Source: CAD feature listing. Evaluate the final solid. Frame: model axes, mm. A direction names the side the tool comes from. Give positions to 0.01 mm unless a question says otherwise; leave off trailing zeros. Loops run counter-clockwise (first coordinate to the right, second up) from the corner with the lowest first, then second, coordinate; pieces in that order, holes last.
```python
from build123d import *

# Parameters (mm, degrees)
F1_DEPTH = 6.35


with BuildPart() as f1:
    # F0 (on Top) → F1 (new body, symmetric)
    with BuildSketch(Plane.XY):
        Polygon((-44.789236, 14.552905), (-40.419224, 17.727905), (-54.301441, 17.727905), (-43.082257, 9.299362), align=None)
        Polygon((-27.68127, -38.1), (-18.27958, -5.362784), (-44.789236, 14.552905), (-43.082257, 9.299362), (-21.934765, -6.587938), (-29.434755, -32.703328), align=None)
        Polygon((-12.292903, 14.552905), (0, 47.09419), (-4.677891, 43.695503), (-14.487496, 17.727905), (-40.419224, 17.727905), (-44.789236, 14.552905), align=None)
        Polygon((-4.677891, 43.695503), (0, 47.09419), (4.677891, 43.695503), (0, 56.078631), align=None)
        Polygon((4.677891, 43.695503), (0, 47.09419), (12.292903, 14.552905), (44.789236, 14.552905), (40.419224, 17.727905), (14.487496, 17.727905), align=None)
        Polygon((54.560881, 17.727905), (40.419224, 17.727905), (44.789236, 14.552905), (43.12004, 9.415647), align=None)
        Polygon((43.12004, 9.415647), (44.789236, 14.552905), (18.49915, -4.547961), (27.68127, -38.1), (29.468066, -32.600809), (22.140832, -5.82664), align=None)
        Polygon((29.468066, -32.600809), (27.68127, -38.1), (22.080786, -38.1), (33.036342, -45.639515), align=None)
        Polygon((27.68127, -38.1), (0, -19.05), (-27.68127, -38.1), (-22.080786, -38.1), (0, -22.904203), (22.080786, -38.1), align=None)
        Polygon((-22.080786, -38.1), (-27.68127, -38.1), (-29.434755, -32.703328), (-33.177816, -45.736876), align=None)
    extrude(amount=F1_DEPTH, both=True)


solid = f1.part
```
(1) Section D-D, the plane x = -24. Return the cut outline in (y, z), then the cut area to 3 significant figures.
A:
outline: (-39.42, -6.35) - (-35.57, -6.35) - (-35.57, 6.35) - (-39.42, 6.35) - close; (-25.28, -6.35) - (-13.78, -6.35) - (-13.78, 6.35) - (-25.28, 6.35) - close; (-5.04, -6.35) - (-1.07, -6.35) - (-1.07, 6.35) - (-5.04, 6.35) - close; (14.55, -6.35) - (17.73, -6.35) - (17.73, 6.35) - (14.55, 6.35) - close
area: 286 mm2
(2) First-contact query: pin 1 (1 mm diameter, centred on y = 22, z = -3.5, fed in from -X); pin 2 (2 mm diameter, centred on x = 42.5, z = -0.5, fed in from +Y). Flat tips, straight axial feed; report the tip coordinate or a pass-through.
A:
pin 1: stops at x = -13.06
pin 2: stops at y = 17.73
(3) Mould query, pull axis Y, two halves, no side actions, for faces 1 (the flat face through (12, 17, -6.35)), 2 (the flat face through (-31.349, 4.456, 0.089)), 3 (the flat face through (35, 17.728, 0)). Classes: pulls with the +Y half, pulls with the -Y half, needs draft (parallel to the pull), parting line crosses it, or undercut.
A:
face 1: needs draft
face 2: undercut
face 3: pulls with the +Y half
(4) Section C-C, the plane y = 6. Return the cut outline in (x, z).
A:
outline: (-38.69, -6.35) - (-33.4, -6.35) - (-33.4, 6.35) - (-38.69, 6.35) - close; (33.02, -6.35) - (38.42, -6.35) - (38.42, 6.35) - (33.02, 6.35) - close
(5) Section A-A, the plane z = -4. Return the cut outline in (x, y).
A:
outline: (-54.3, 17.73) - (-21.93, -6.59) - (-33.18, -45.74) - (0, -22.9) - (33.04, -45.64) - (22.14, -5.83) - (54.56, 17.73) - (14.49, 17.73) - (0, 56.08) - (-14.49, 17.73) - close; hole (-44.79, 14.55) - (-18.28, -5.36) - (-27.68, -38.1) - (0, -19.05) - (27.68, -38.1) - (18.5, -4.55) - (44.79, 14.55) - (12.29, 14.55) - (0, 47.09) - (-12.29, 14.55) - close
(6) Reachability of faces 4 (the flat face through (12, 17, 6.35)), 5 (the flat face through (-34, 17.728, 0)), 6 (the flat face through (-23.046, -21.961, 0.089)) from +Z, -Z, +X, -X, +Y, -Y: full face, straight path, thin tool, end or side. Return the list, or none.
A:
face 4: +Z, +X, -X, +Y, -Y
face 5: +Z, -Z, -X, +Y
face 6: +Z, -Z
(7) Ray query, line 1 along X through (y, z) = (-28, -1.25); line 2 along X through (y, z) = (-25.5, 2); line 3 along X through (y, z) = (9, -1). Return the intervals inside material, ascending.
A:
line 1: x = -28.08 to -24.78, -13.01 to -7.4, 7.4 to 13.01, 24.92 to 28.21
line 2: x = -27.37 to -24.06, -9.37 to -3.77, 3.77 to 9.37, 24.23 to 27.52
line 3: x = -42.68 to -37.4, 37.15 to 42.55
(8) Section B-B, the plane x = -36. Return the cut outline in (y, z).
A:
outline: (3.98, -6.35) - (7.95, -6.35) - (7.95, 6.35) - (3.98, 6.35) - close; (14.55, -6.35) - (17.73, -6.35) - (17.73, 6.35) - (14.55, 6.35) - close
